Part model, mm, in its own coordinate system. A direction names the side the tool comes from. Round coordinates to 2 decimals unless told otherwise and drop trailing zeros. Write each loop counter-clockwise with the first axis right and the second up, starting at its lowest first coordinate (ties: lowest second). Pieces come first, ordered by that corner, then holes.
1) Saw through at D-D on z = 157.5. Write the cut outline in (x, y), and give its area (3 significant figures).
2) Pull direction X, two halves, no side cores. Call faces 3 (the cylindrical face through (-90.07, 28.91, 164.25)), 4 (the flat face through (-63.234, 20, 175)), 5 (the cylindrical face through (-75.218, 3.863, 187.323)): +X half, -X half, draft (parallel to the pull), parting line (faces both ways), or undercut.
3) Which spindle directions (+Z, -Z, +X, -X, +Y, -Y) get a long thin tool onto all of the face, cutting with end or side? Do faces 1 (the flat face through (-89, 0, 168)), 2 (the flat face through (-89, 7.62, 174)). Say none if no direction does.
4) Saw through at B-B on y = 44. Write the cut outline in (x, z) (3 decimals).
5) Saw through at C-C on x = -77. Write the cut outline in (y, z), and give its area (3 significant figures).
6) Saw through at A-A on x = -100. Write the cut outline in (y, z).
7) Flat gauge pins, fed straight in: pin 1 (6 mm diameter, centred on x = -79, y = 28.5, fed in from +Z); pin 2 (4 mm diameter, centred on y = 26, z = 169.5, fed in from -X); pin 3 (3 mm diameter, centred on y = 14.5, z = 149.5, fed in from +X); pin 4 (4.5 mm diameter, centred on x = -101.33, z = 172.46, fed in from -Y). Where does each tip first touch, or does it go through?
8) Drill centre lines: L1, parallel to Y at x = -78, z = 192; L2, parallel to Z at x = -75.5, y = 4.5; L3, parallel to Z at x = -90.5, y = 14. Where is each one in solid material? Low to high.
```python
from build123d import *

# Parameters (mm, degrees)
BOSS_EXTRUDE1_DEPTH = 50.8
CUT_EXTRUDE1_START  = -43.18
SKETCH2_R           = 209.55
SKETCH2_R_2         = 187.325
CUT_EXTRUDE1_DEPTH  = 43.18
SKETCH3_R           = 2.38125
CUT_EXTRUDE2_DEPTH  = 43.18


with BuildPart() as part:
    # Sketch1 → Boss-Extrude1 (new body)
    with BuildSketch(Plane(origin=(0, 0, 0), x_dir=(1, 0, 0), z_dir=(0, 1, 0))):
        with BuildLine():
            Line((-63.233720515, -199.781628509), (-63.233720515, -167.533762239))
            ThreePointArc((-63.233720515, -167.533762239), (-89.849960422, -154.896899621), (-114.033720515, -138.066561793))
            Line((-114.033720515, -138.066561793), (-114.033720515, -175.805327239))
            ThreePointArc((-114.033720515, -175.805327239), (-89.440774639, -189.503430924), (-63.233720515, -199.781628509))
        make_face()
    extrude(amount=BOSS_EXTRUDE1_DEPTH)

    # Sketch2 → Cut-Extrude1 (cut)
    with BuildSketch(Plane(origin=(0, 50.8, 0), x_dir=(1, 0, 0), z_dir=(0, 1, 0)).offset(CUT_EXTRUDE1_START)):
        Circle(SKETCH2_R)
        Circle(SKETCH2_R_2, mode=Mode.SUBTRACT)
    extrude(amount=CUT_EXTRUDE1_DEPTH, mode=Mode.SUBTRACT)

    # Sketch3 → Cut-Extrude2 (cut)
    with BuildSketch(Plane(origin=(0, 7.62, 0), x_dir=(1, 0, 0), z_dir=(0, 1, 0))):
        with Locations(Location((-101.333720515, -172.457176457, 0), (0, 0, 270))):
            Circle(SKETCH3_R)
        with Locations(Location((-75.933720515, -185.051535291, 0), (0, 0, 270))):
            Circle(SKETCH3_R)
    extrude(amount=-CUT_EXTRUDE2_DEPTH, mode=Mode.SUBTRACT)


solid = part.part
```
Completed:
1. outline: (-114.03, 0) - (-85.2, 0) - (-85.2, 50.8) - (-101.41, 50.8) - (-101.41, 7.62) - (-114.03, 7.62) - close
1. area: 920 mm2
2. face 3: -X half
2. face 4: +X half
2. face 5: undercut
3. face 1: +Z, -Z, +X, -X, -Y
3. face 2: +Z, -X, +Y
4. outline: (-114.034, 138.067) arc R179.07 cw to (-63.234, 167.534) - (-63.234, 176.33) arc R187.325 ccw to (-114.034, 148.617) - close
5. outline: (0, 161.67) - (50.8, 161.67) - (50.8, 170.77) - (7.62, 170.77) - (7.62, 182.92) - (0, 182.92) - close; (0, 187.18) - (7.62, 187.18) - (7.62, 194.89) - (0, 194.89) - close
5. area: 614 mm2
6. outline: (0, 148.55) - (50.8, 148.55) - (50.8, 158.4) - (7.62, 158.4) - (7.62, 170.48) - (0, 170.48) - close; (0, 174.43) - (7.62, 174.43) - (7.62, 184.15) - (0, 184.15) - close
7. pin 1: stops at z = 171.22
7. pin 2: stops at x = -83.87
7. pin 3: stops at x = -96.26
7. pin 4: passes through
8. L1: y = 0 to 7.62
8. L2: z = 162.38 to 182.71, 187.39 to 195.48
8. L3: z = 154.52 to 164.01
